Design review of the part built by this model. Coordinates are the model's own, in mm. Face numbers are marked on the shaded views. A direction names the side the tool comes from. Coordinates: 2 decimals unless noted, no trailing zeros. Loops run counter-clockwise (first coordinate to the right, second up) from the corner with the lowest first, then second, coordinate; pieces in that order, holes last.
from build123d import *

# Parameters (mm, degrees)
BOSS_EXTRUDE1_DEPTH = 4.7625
FILLET1_R           = 9.525
FILLET2_R           = 1.5875
FILLET4_R           = 12.7
SKETCH2_W           = 6.35
SKETCH2_H           = 6.35
BOSS_EXTRUDE2_DEPTH = 4.7625


with BuildPart() as part:
    # Sketch1 → Boss-Extrude1 (new body)
    with BuildSketch(Plane(origin=(0, 0, 0), x_dir=(1, 0, 0), z_dir=(0, 1, 0))):
        with BuildLine():
            ThreePointArc((62.2046, 11.1252), (55.805583, 0.025067), (42.993099, 0))
            Line((42.993099, 0), (3.175, 0))
            Line((3.175, 0), (20.9296, -9.525))
            Line((20.9296, -9.525), (62.2046, -9.525))
            Line((62.2046, -9.525), (62.2046, 11.1252))
        make_face()
    extrude(amount=BOSS_EXTRUDE1_DEPTH)

    # Fillet1
    fillet1_edges = [part.edges().sort_by_distance(p)[0] for p in [
        (62.2046, 2.38125, 9.525),
    ]]
    fillet(fillet1_edges, radius=FILLET1_R)

    # Fillet2
    fillet2_edges = [part.edges().sort_by_distance(p)[0] for p in [
        (62.2046, 2.38125, -11.1252),
    ]]
    fillet(fillet2_edges, radius=FILLET2_R)

    # Fillet4
    fillet4_edges = [part.edges().sort_by_distance(p)[0] for p in [
        (20.9296, 2.38125, 9.525),
    ]]
    fillet(fillet4_edges, radius=FILLET4_R)

    # Sketch2 → Boss-Extrude2 (add)
    with BuildSketch(Plane.XZ):
        with Locations((24.0645, -3.175)):
            Rectangle(SKETCH2_W, SKETCH2_H)
    extrude(amount=-BOSS_EXTRUDE2_DEPTH)


solid = part.part
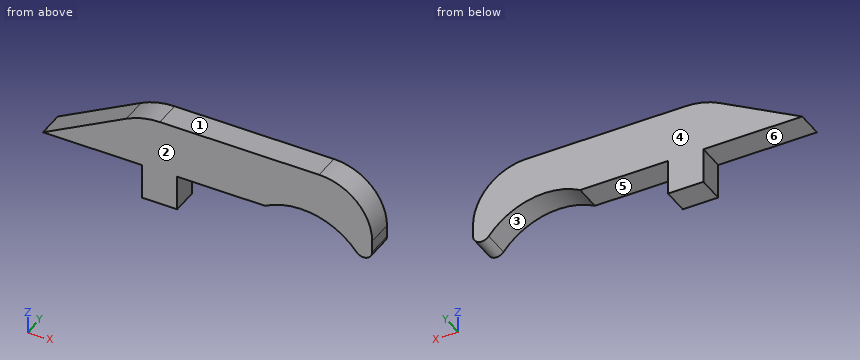
Q1. Take a section at C-C, the plane x = 34.5. Write out the cut boundary in (y, z) (1 decimal), then the cut area to 3 significant figures.
Q2. Machinability: for the marked faces 4, 5 and 6, which of the approach directions +Z, -Z, +X, -X, +Y, -Y give a long, thin tool a straight path to every point of the face, cutting with its end or side? Answer none if there is none.
Q3. The part is to be moulded in two halves that separate along Z. For the marked faces 1, 2 and 3, say which applies: pulls with the +Z half, pulls with the -Z half, needs draft (parallel to the pull), parting line crosses it, or undercut.
Q4. For line 1 (Z direction, x = 31.5, y = 4.2) (3 decimals); line 2 (X direction, y = 1.25, z = -5); line 3 (Z direction, x = 56, y = 3.5), list the stretches that pass through material, from the lowest coordinate up.
Q5. Take a section at A-A, the plane z = 0.5. Write out the cut boundary in (x, y), then the cut area to 3 significant figures.
Q6. Clearance check with a flat-ended pin moving along its axis: pin 1 Ø1.4 at (x, y) = (33.5, 1.5) entering from -Z. State where the tip first meets the part, or that it passes through.
Q7. Take a section at D-D, the plane z = -4.5. Write out the cut boundary in (x, y).
Entries:
1. outline: (0, 0) - (4.8, 0) - (4.8, 9.5) - (0, 9.5) - close
1. area: 45.4 mm2
2. face 4: +Z, -Z, +X, -X, +Y
2. face 5: -Z, +Y, -Y
2. face 6: -Z, -X, +Y, -Y
3. face 1: pulls with the +Z half
3. face 2: needs draft
3. face 3: pulls with the -Z half
4. line 1: z = 0 to 9.525
4. line 2: x = 20.89 to 27.24
4. line 3: z = -0.14 to 8.93
5. outline: (4.11, 0) - (43.96, 0) - (43.96, 4.76) - (4.11, 4.76) - close; (54.8, 0) - (62.19, 0) - (62.19, 4.76) - (54.8, 4.76) - close
5. area: 225 mm2
6. pin 1: stops at z = 0
7. outline: (20.89, 0) - (27.24, 0) - (27.24, 4.76) - (20.89, 4.76) - close
